Can you work these out from the model? Positions are in its coordinate system, mm. A direction names the side the tool comes from. Give positions to 0.01 mm unless a question says otherwise; leave off trailing zeros. Write each loop counter-clockwise with the first axis right and the second up, starting at its lowest first coordinate (ties: lowest second). Pieces come first, ordered by that corner, then holes. Notation, with made-up numbers: (0, 42.25) -> (10, 42.25) arc R20 cw to (10, 68.25) -> close; hole circle Ø2 at (-21.75, -28.75). An arc over 180 degrees is marked (long way). Answer as CSV lines item,"result". Start each with the question number.
1. If we section it at A-A on x = -19.05: Write out the boundary of the cut face in (y, z), plus the area to 3 significant figures.
2. If we section it at C-C on x = -30: Write out the boundary of the cut face in (y, z).
3. I'm going to push flat-ended pins straight in: P1, Ø8, axis at x = -33.5, y = -24, coming from the -Z side; P2, Ø1, axis at y = -19.5, z = -43.5, coming from the -X side; P3, Ø2, axis at y = -14, z = -21, coming from the -X side. Where does each tip first touch, or does it pass through?
4. I need wall thicknesses on line 1 (Y direction, x = -19, z = -2); line 2 (Z direction, x = -19, y = -13.5); line 3 (X direction, y = -19, z = -2). Which ranges of each line are inside material? Lowest first, please. Write a range as [from, to].
5. If we mould it in two halves opening along Y, with no side actions, what happens to faces 3 (the face through (-23, -19, 0)), 4 (the face through (-23, -38.1, -2)), 5 (the face through (-20.7, -19, -1.6)), 6 (the face through (-42.263, -18.732, -26.482))? For each: pulls with the +Y half, pulls with the -Y half, needs draft (parallel to the pull), parting line crosses it, or undercut.
6. On a 3-axis mill with a long thin cutter (end or side, diameter ignored), from which of +Z, -Z, +X, -X, +Y, -Y can I reach the whole of each face in a straight line? I mean faces 1 (the face through (0, -19, -2)), 2 (the face through (-23, -19, -3.302)). Say none if no direction works.
7. If we section it at B-B on z = -45.5: Write out the boundary of the cut face in (x, y), plus the area to 3 significant figures.
```python
from build123d import *

# Parameters (mm, degrees)
SKETCH13_R              = 1.651
BASE_FLANGE5_DEPTH      = 3.302
EDGE_FLANGE4_START      = -51.763631849
EDGE_FLANGE4_DEPTH      = 40.665312179
CUT_EXTRUDE4_DEPTH      = 4.699
CUT_EXTRUDE4_DEPTH_BACK = 56.896


# Read off the part's stored shape, not the designer's step: Edge-Flange4
# Sheet-metal steps are written as plain solids
with BuildPart() as part:
    # Sketch13 → Base-Flange5 (new body)
    with BuildSketch(Plane.XY):
        Polygon((-31.75, 0), (0, 0), (0, -38.1), (-45.964697135, -38.1), align=None)
        with Locations((-19.05, -19.05)):
            Circle(SKETCH13_R, mode=Mode.SUBTRACT)
    extrude(amount=-BASE_FLANGE5_DEPTH)

    # Edge-Flange4 outline → Edge-Flange4 (add)
    with BuildSketch(Plane(origin=(0, 0, 0), x_dir=(0.9369164518419233, -0.34955337542060905, 0), z_dir=(0.34955337542060905, 0.9369164518419232, 0)).offset(EDGE_FLANGE4_START)):
        with BuildLine():
            ThreePointArc((-33.049097346, 3.302), (-32.081963937, 0.967133409), (-29.747097346, 0))
            Line((-29.747097346, 0), (-29.747097346, 49.022))
            Line((-29.747097346, 49.022), (-33.049097346, 49.022))
            Line((-33.049097346, 49.022), (-33.049097346, 3.302))
        make_face()
    extrude(amount=EDGE_FLANGE4_DEPTH)

    # Sketch51 → Cut-Extrude4 (cut, two sides: drawn at the far end of the back side and taken through both)
    with BuildSketch(Plane.XY.offset(-CUT_EXTRUDE4_DEPTH_BACK)):
        Polygon((-31.75, 0), (-35.274327056, 0), (-34.843698124, 1.154225246), align=None)
    extrude(amount=CUT_EXTRUDE4_DEPTH + CUT_EXTRUDE4_DEPTH_BACK, mode=Mode.SUBTRACT)


solid = part.part
```
Computed values:
1,outline,"(-38.1, -3.3) -> (-20.7, -3.3) -> (-20.7, 0) -> (-38.1, 0) -> close; (-17.4, -3.3) -> (0, -3.3) -> (0, 0) -> (-17.4, 0) -> close"
1,area,"115 mm2"
2,outline,"(-38.1, -3.3) -> (0, -3.3) -> (0, 0) -> (-38.1, 0) -> close"
3,P1,"stops at z = -3.3"
3,P2,"stops at x = -42.74"
3,P3,"stops at x = -40.87"
4,line 1,"y = [-38.1, -20.7], [-17.4, 0]"
4,line 2,"z = [-3.3, 0]"
4,line 3,"x = [-42.08, -20.7], [-17.4, 0]"
5,face 3,"needs draft"
5,face 4,"pulls with the -Y half"
5,face 5,"undercut"
5,face 6,"pulls with the +Y half"
6,face 1,"+Z, -Z, +X, +Y, -Y"
6,face 2,"-Z, +X, -Y"
7,outline,"(-49.06, -36.95) -> (-45.96, -38.1) -> (-31.75, 0) -> (-35.27, 0) -> close"
7,area,"132 mm2"
